Part model, mm, in its own coordinate system. Face numbers are marked on the shaded views. A direction names the side the tool comes from. Round coordinates to 2 decimals unless told otherwise and drop trailing zeros. Loops run counter-clockwise (first coordinate to the right, second up) from the corner with the lowest first, then second, coordinate; pieces in that order, holes last. Notation, with made-up numbers: (-16.75, 89) -> (28.25, 89) arc R9 cw to (28.25, 97) -> close; hole circle Ø6 at (-28.75, -7). An arc over 180 degrees is marked (long way). Use a Markdown table: item, result. Add a question column.
Item 1: Cut at B-B, the plane z = -1. List the corners of the cut face in (x, y) (3 decimals).
Item 2: Flat gauge pins, fed straight in: pin 1 (4 mm diameter, centred on y = 24.5, z = 1, fed in from -X) (3 decimals); pin 2 (5 mm diameter, centred on y = 23, z = 41.5, fed in from +X); pin 3 (5 mm diameter, centred on y = 19.5, z = 22.5, fed in from -X) (3 decimals). Where does each tip first touch, or does it go through?
Item 3: Which spindle directions (+Z, -Z, +X, -X, +Y, -Y) get a long thin tool onto all of the face, cutting with end or side? Do the marked faces 1, 2, 3, 4 and 5. Say none if no direction does.
Item 4: Cut at A-A, the plane y = -50. List the corners of the cut face in (x, z) (3 decimals).
Item 5: Probe line 1 (Z direction, x = 66.5, y = 7) (3 decimals); line 2 (X direction, y = -33, z = 4) (3 decimals); line 3 (Z direction, x = -6.5, y = -9) (3 decimals). List the from-to ranges inside material, lowest first. Write a range as [from, to].
```python
from build123d import *

# Parameters (mm, degrees)
F1_DEPTH = 63.5
F2_DEPTH = 25.4
F3_DEPTH = 7.9375
F0_W     = 25.4
F0_H     = 4.7498
F0_H_2   = 19.05
F0_H_3   = 4.7752


# Not quite as in the source:
# - a feature names something its author has since deleted; it is built from what else it names


with BuildPart() as f1:
    # F0 (on Front) → F1 (new body, symmetric)
    with BuildSketch(Plane.XZ):
        Polygon((-41.275, -9.525), (41.275, -9.525), (41.275, 9.525), (22.225, 9.525), (-41.275, 9.525), align=None)
    extrude(amount=F1_DEPTH, both=True)

    # F0 (on Front) → F2 (join, symmetric)
    with BuildSketch(Plane.XZ):
        with BuildLine():
            Line((22.225, 9.525), (41.275, 9.525))
            Line((41.275, 9.525), (41.275, 27.0002))
            ThreePointArc((41.275, 27.0002), (45.9246798487, 38.2255201513), (57.15, 42.8752))
            Line((57.15, 42.8752), (60.325, 42.8752))
            Line((60.325, 42.8752), (60.325, 61.9252))
            Line((60.325, 61.9252), (57.15, 61.9252))
            ThreePointArc((57.15, 61.9252), (32.4542956671, 51.6959043329), (22.225, 27.0002))
            Line((22.225, 27.0002), (22.225, 9.525))
        make_face()
    extrude(amount=F2_DEPTH, both=True)

    # F0 (on Front) → F3 (join, symmetric)
    with BuildSketch(Plane.XZ):
        with BuildLine():
            add(Edge.make_bspline(
                [(-41.275, 9.525), (-41.7312111626, 19.5100846971), (-7.2445928525, 66.0155981062), (57.15, 61.9252)],
                knots=[0, 0, 0, 0, 111.5045361635, 111.5045361635, 111.5045361635, 111.5045361635], degree=3))
            Line((-41.275, 9.525), (22.225, 9.525))
            Line((22.225, 9.525), (22.225, 27.0002))
            ThreePointArc((22.225, 27.0002), (32.4542956671, 51.6959043329), (57.15, 61.9252))
        make_face()
    extrude(amount=F3_DEPTH, both=True)

    # F0 (on Front) → F4 (revolve)
    with BuildSketch(Plane.XZ):
        with Locations((73.025, 64.3001)):
            Rectangle(F0_W, F0_H)
        with Locations((73.025, 52.4002)):
            Rectangle(F0_W, F0_H_2)
        with Locations((73.025, 40.4876)):
            Rectangle(F0_W, F0_H_3)
    revolve(axis=Axis((60.325, 0, 52.3875), (0, 0, 1)))


solid = f1.part
```
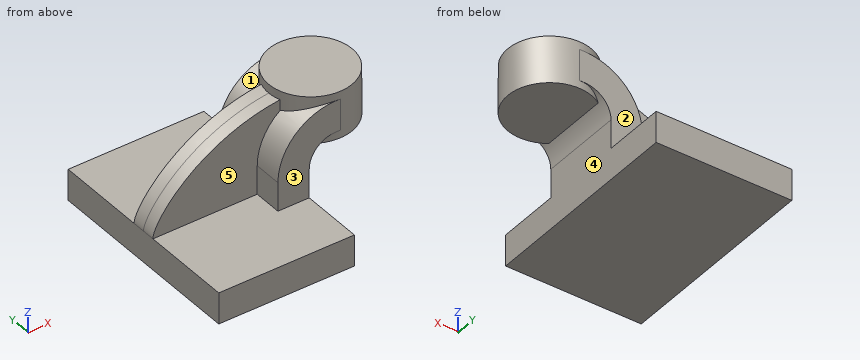
A:
| question | item | result |
|---|---|---|
| 1 | outline | (-41.275, -63.5) -> (41.275, -63.5) -> (41.275, 63.5) -> (-41.275, 63.5) -> close |
| 2 | pin 1 | stops at x = -41.275 |
| 2 | pin 2 | stops at x = 75.32 |
| 2 | pin 3 | stops at x = 22.225 |
| 3 | face 1 | +Z, -X, +Y |
| 3 | face 2 | +Z, +X, -X, +Y |
| 3 | face 3 | +Z, +X, -X, -Y |
| 3 | face 4 | -Z, +X, +Y, -Y |
| 3 | face 5 | +Z, -X, -Y |
| 4 | outline | (-41.275, -9.525) -> (41.275, -9.525) -> (41.275, 9.525) -> (-41.275, 9.525) -> close |
| 5 | line 1 | z = [38.1, 66.675] |
| 5 | line 2 | x = [-41.275, 41.275] |
| 5 | line 3 | z = [-9.525, 9.525] |
